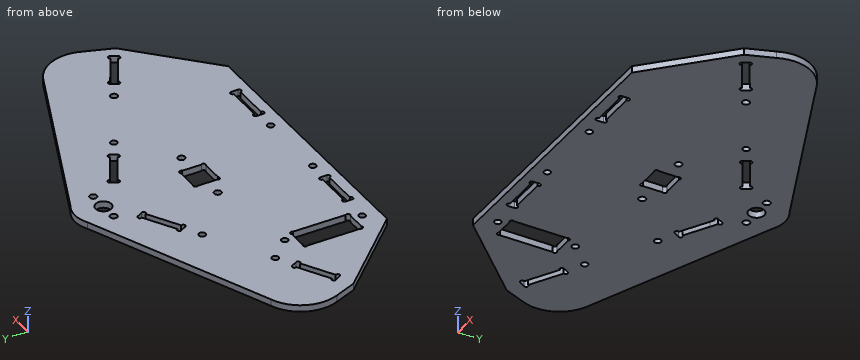
```python
from build123d import *

# Parameters (mm, degrees)
MODEL_R             = 3.781579339
MODEL_R_2           = 1.7
MODEL_R_3           = 1.6
MODEL_W             = 12
MODEL_H             = 28
MODEL_W_2           = 13
MODEL_H_2           = 12
BOSS_EXTRUDE2_DEPTH = 3.2
SKETCH1_R           = 1.0005
CUT_EXTRUDE1_DEPTH  = 312.966216485


with BuildPart() as part:
    # Model → Boss-Extrude2 (new body)
    with BuildSketch(Plane.XY):
        with BuildLine():
            Line((88, 60), (220, 60))
            Line((220, 60), (254.882583618, 93.640518188))
            Line((254.882583618, 93.640518188), (259.489592216, 106.576108559))
            ThreePointArc((259.489592216, 106.576108559), (259.424141413, 121.57623231), (248.498382723, 131.854159795))
            Line((248.498382723, 131.854159795), (161.617078665, 168.980084934))
            ThreePointArc((161.617078665, 168.980084934), (154.617078665, 170.855729281), (147.617078665, 168.980084934))
            Line((147.617078665, 168.980084934), (59.501617277, 131.854159795))
            ThreePointArc((59.501617277, 131.854159795), (48.575858587, 121.57623231), (48.510407784, 106.576108559))
            Line((48.510407784, 106.576108559), (52.677086204, 96.362955936))
            Line((52.677086204, 96.362955936), (88, 60))
        make_face()
        with Locations((154.617078665, 157.237991333)):
            Circle(MODEL_R, mode=Mode.SUBTRACT)
        with Locations((163.114624023, 157.237991333)):
            Circle(MODEL_R_2, mode=Mode.SUBTRACT)
        with Locations((146.117078665, 157.237991333)):
            Circle(MODEL_R_2, mode=Mode.SUBTRACT)
        with Locations((115.877120948, 132.296819167)):
            Circle(MODEL_R_3, mode=Mode.SUBTRACT)
        with Locations((137.734977924, 66.871509225)):
            Circle(MODEL_R_3, mode=Mode.SUBTRACT)
        with Locations((193.918561918, 129.673741782)):
            Circle(MODEL_R_3, mode=Mode.SUBTRACT)
        with Locations((172.735008, 66.871509225)):
            Circle(MODEL_R_3, mode=Mode.SUBTRACT)
        with Locations((170.033762, 111.08294)):
            Circle(MODEL_R_2, mode=Mode.SUBTRACT)
        with Locations((140, 111)):
            Circle(MODEL_R_2, mode=Mode.SUBTRACT)
        with Locations((95.2, 104.75)):
            Circle(MODEL_R_3, mode=Mode.SUBTRACT)
        with Locations((85.560630532, 114.806524888)):
            Circle(MODEL_R_3, mode=Mode.SUBTRACT)
        with Locations((224.233700932, 112.158328537)):
            Circle(MODEL_R_2, mode=Mode.SUBTRACT)
        with Locations((95.2, 67.75)):
            Circle(MODEL_R_3, mode=Mode.SUBTRACT)
        with Locations((93, 86)):
            Rectangle(MODEL_W, MODEL_H, mode=Mode.SUBTRACT)
        Polygon((181.734462562, 65.257395619), (181.735489, 68.457395619), (202.735488, 68.450659619), (202.734461562, 65.250659619), align=None, mode=Mode.SUBTRACT)
        Polygon((249.399348556, 95.770313962), (231.216181373, 106.276143646), (232.817069658, 109.046911896), (251.000236841, 98.541082213), align=None, mode=Mode.SUBTRACT)
        Polygon((60.374623433, 98.42894725), (58.775510803, 101.200740676), (76.965405371, 111.694917426), (78.564518, 108.923124), align=None, mode=Mode.SUBTRACT)
        Polygon((128.734464562, 65.274396), (128.735491, 68.474396), (107.735493, 68.481132), (107.734466562, 65.281132), align=None, mode=Mode.SUBTRACT)
        Polygon((142.66224045, 145.902603249), (124.4723462, 135.408426681), (122.873233571, 138.180220108), (136.035908619, 145.774076024), (141.063127638, 148.674396991), align=None, mode=Mode.SUBTRACT)
        Polygon((167.142166, 143.296685), (168.743054285, 146.067453251), (186.926220285, 135.561624251), (185.325332, 132.790856), align=None, mode=Mode.SUBTRACT)
        with Locations((155.035687, 111.089836)):
            Rectangle(MODEL_W_2, MODEL_H_2, mode=Mode.SUBTRACT)
    extrude(amount=BOSS_EXTRUDE2_DEPTH)

    # Sketch1 → Cut-Extrude1 (cut, through all)
    with BuildSketch(Plane.XY.offset(3.2)):
        with Locations((61.241241971, 98.928919808)):
            Circle(SKETCH1_R)
        with Locations((59.642129342, 101.700713234)):
            Circle(SKETCH1_R)
        with Locations((76.098786832, 111.194944868)):
            Circle(SKETCH1_R)
        with Locations((77.697899462, 108.423151442)):
            Circle(SKETCH1_R)
        with Locations((87.707460335, 99.292539665)):
            Circle(SKETCH1_R)
        with Locations((98.292539665, 99.292539665)):
            Circle(SKETCH1_R)
        with Locations((87.707460335, 72.707460335)):
            Circle(SKETCH1_R)
        with Locations((98.292539665, 72.707460335)):
            Circle(SKETCH1_R)
        with Locations((108.735992948, 68.480811078)):
            Circle(SKETCH1_R)
        with Locations((108.73496651, 65.280811078)):
            Circle(SKETCH1_R)
        with Locations((127.733964613, 65.274716923)):
            Circle(SKETCH1_R)
        with Locations((127.734991051, 68.474716923)):
            Circle(SKETCH1_R)
        with Locations((182.73496251, 65.257074697)):
            Circle(SKETCH1_R)
        with Locations((182.735988949, 68.457074697)):
            Circle(SKETCH1_R)
        with Locations((201.734988051, 68.450980541)):
            Circle(SKETCH1_R)
        with Locations((201.733961613, 65.250980541)):
            Circle(SKETCH1_R)
        with Locations((232.082479384, 105.775615918)):
            Circle(SKETCH1_R)
        with Locations((233.683367669, 108.546384168)):
            Circle(SKETCH1_R)
        with Locations((250.13393883, 99.041609941)):
            Circle(SKETCH1_R)
        with Locations((248.533050545, 96.27084169)):
            Circle(SKETCH1_R)
        with Locations((160.828226665, 105.797296335)):
            Circle(SKETCH1_R)
        with Locations((160.828226665, 116.382375665)):
            Circle(SKETCH1_R)
        with Locations((149.243147335, 105.797296335)):
            Circle(SKETCH1_R)
        with Locations((149.243147335, 116.382375665)):
            Circle(SKETCH1_R)
        with Locations((168.008464011, 142.796157272)):
            Circle(SKETCH1_R)
        with Locations((169.609352296, 145.566925523)):
            Circle(SKETCH1_R)
        with Locations((184.459033989, 133.291383728)):
            Circle(SKETCH1_R)
        with Locations((186.059922274, 136.062151978)):
            Circle(SKETCH1_R)
        with Locations((141.795621912, 145.402630691)):
            Circle(SKETCH1_R)
        with Locations((140.196509099, 148.174424012)):
            Circle(SKETCH1_R)
        with Locations((123.739852109, 138.680192666)):
            Circle(SKETCH1_R)
        with Locations((125.338964739, 135.90839924)):
            Circle(SKETCH1_R)
    extrude(amount=-CUT_EXTRUDE1_DEPTH, mode=Mode.SUBTRACT)


solid = part.part
```
Here's how the part is built. I have some questions about the finished solid (model axes, mm). Coordinates: 2 decimals unless noted, no trailing zeros. Return JSON: item names as keys, results as strings.
1) If I drill on probe 1 along Y at (x, z) = (95.2, 1.05); probe 2 along Y at (x, z) = (173, 2.9); probe 3 along X at (y, z) = (66, 1.1), over which ranges is the centre line in solid material (lowest first)?
Conclusion:
{"probe 1": "y = 60 to 66.15, 69.35 to 72, 100 to 103.15, 106.35 to 146.9", "probe 2": "y = 60 to 65.29, 68.45 to 139.91, 143.61 to 164.12", "probe 3": "x = 82.17 to 107.73, 128.73 to 136.39, 139.08 to 171.39, 174.08 to 181.73, 202.73 to 226.22"}
2) I'm going to push flat-ended pins straight in: P1, Ø1, axis at x = 134.5, z = 1, coming from the +Y side; P2, Ø1, axis at y = 113, z = 2.5, coming from the -X side; P3, Ø1.6, axis at y = 89, z = 1.5, coming from the +X side. Where does each tip first touch, or does it pass through?
Conclusion:
{"P1": "stops at y = 163.66", "P2": "stops at x = 47.01", "P3": "stops at x = 250.9"}
3) If we section it at A-A on z = 1.2: State how many separate pieces and enclosed holes the cut face has, plus the area to 3 significant figures.
Conclusion:
{"separate pieces": "1", "enclosed holes": "21", "area": "16,200 mm²"}
